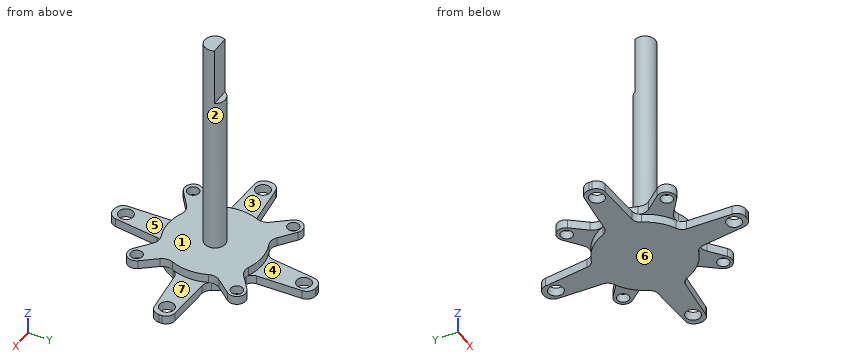
from build123d import *

# Parameters (mm, degrees)
SKETCH_2_R          = 3.5
EXTRUDE_1_DEPTH     = 75
SKETCH_3_R          = 2
EXTRUDE_2_DEPTH     = 3
FILLET_1_R          = 5
SKETCH_5_R          = 16
EXTRUDE_3_DEPTH     = 3
FILLET_2_R          = 4
SKETCH_6_R          = 2.5
EXTRUDE_4_DEPTH     = 3
FILLET_3_R          = 3
FILLET_4_R          = 3
CUT_EXTRUDE_1_DEPTH = 20


with BuildPart() as part:
    # 草图2 → 凸台-拉伸1 (new body)
    with BuildSketch(Plane.XY):
        Circle(SKETCH_2_R)
    extrude(amount=-EXTRUDE_1_DEPTH)

    # 草图3 → 凸台-拉伸2 (add)
    with BuildSketch(Plane(origin=(0, 0, -75), x_dir=(-1, 0, 0), z_dir=(0, 0, -1))):
        with BuildLine():
            Line((-19.333172355, 15.121758852), (-7.5, 0))
            Line((-7.5, 0), (-19.333172355, -15.121758852))
            ThreePointArc((-19.333172355, -15.121758852), (-19.091883092, -19.091883092), (-15.121758852, -19.333172355))
            Line((-15.121758852, -19.333172355), (0, -7.5))
            Line((0, -7.5), (15.407660085, -19.397223244))
            ThreePointArc((15.407660085, -19.397223244), (19.379165256, -19.127226562), (19.586420792, -15.151953404))
            Line((19.586420792, -15.151953404), (7.5, 0))
            Line((7.5, 0), (19.586420792, 15.151953404))
            ThreePointArc((19.586420792, 15.151953404), (19.379165256, 19.127226562), (15.407660085, 19.397223244))
            Line((15.407660085, 19.397223244), (0, 7.5))
            Line((0, 7.5), (-15.121758852, 19.333172355))
            ThreePointArc((-15.121758852, 19.333172355), (-19.091883092, 19.091883092), (-19.333172355, 15.121758852))
        make_face()
        with Locations((-16.970562748, 16.970562748)):
            Circle(SKETCH_3_R, mode=Mode.SUBTRACT)
        with Locations((16.970562748, 16.970562748)):
            Circle(SKETCH_3_R, mode=Mode.SUBTRACT)
        with Locations((16.970562748, -16.970562748)):
            Circle(SKETCH_3_R, mode=Mode.SUBTRACT)
        with Locations((-16.970562748, -16.970562748)):
            Circle(SKETCH_3_R, mode=Mode.SUBTRACT)
    extrude(amount=EXTRUDE_2_DEPTH)

    # 圆角1
    fillet_1_edges = [part.edges().sort_by_distance(p)[0] for p in [
        (7.5, 0, -76.5),
        (0, -7.5, -76.5),
        (-7.5, 0, -76.5),
        (0, 7.5, -76.5),
    ]]
    fillet(fillet_1_edges, radius=FILLET_1_R)

    # 草图5 → 凸台-拉伸3 (add)
    with BuildSketch(Plane.XY.offset(-75)):
        Circle(SKETCH_5_R)
    extrude(amount=-EXTRUDE_3_DEPTH)

    # 圆角2
    fillet_2_edges = [part.edges().sort_by_distance(p)[0] for p in [
        (8.070562783, -13.815426753, -76.5),
        (13.815426753, -8.070562783, -76.5),
        (-8.132091519, -13.779299239, -76.5),
        (-13.866910674, -7.981778521, -76.5),
        (-13.866910674, 7.981778521, -76.5),
        (-8.132091519, 13.779299239, -76.5),
        (8.070562783, 13.815426753, -76.5),
        (13.815426753, 8.070562783, -76.5),
    ]]
    fillet(fillet_2_edges, radius=FILLET_2_R)

    # 草图6 → 凸台-拉伸4 (add)
    with BuildSketch(Plane(origin=(0, 0, -78), x_dir=(-1, 0, 0), z_dir=(0, 0, -1))):
        with BuildLine():
            Line((-4.536268833, 32.087497482), (-5.241257707, 15.117182861))
            ThreePointArc((-5.241257707, 15.117182861), (-11.313708499, 11.313708499), (-15.117182861, 5.241257707))
            Line((-15.117182861, 5.241257707), (-32.087497482, 4.536268833))
            ThreePointArc((-32.087497482, 4.536268833), (-34.077297457, 3.667151814), (-34.959506593, 1.683121729))
            ThreePointArc((-34.959506593, 1.683121729), (-34.979209977, 1.206179654), (-34.992406887, 0.729013218))
            ThreePointArc((-34.992406887, 0.729013218), (-34.248960415, -1.311073956), (-32.323754723, -2.31519117))
            Line((-32.323754723, -2.31519117), (-15.442311817, -4.187482029))
            ThreePointArc((-15.442311817, -4.187482029), (-11.313708499, -11.313708499), (-4.187482029, -15.442311817))
            Line((-4.187482029, -15.442311817), (-2.31519117, -32.323754723))
            ThreePointArc((-2.31519117, -32.323754723), (-1.311073956, -34.248960415), (0.729013218, -34.992406887))
            ThreePointArc((0.729013218, -34.992406887), (1.206179654, -34.979209977), (1.683121729, -34.959506593))
            ThreePointArc((1.683121729, -34.959506593), (3.667151814, -34.077297457), (4.536268833, -32.087497482))
            Line((4.536268833, -32.087497482), (5.241257707, -15.117182861))
            ThreePointArc((5.241257707, -15.117182861), (11.313708499, -11.313708499), (15.117182861, -5.241257707))
            Line((15.117182861, -5.241257707), (32.087497482, -4.536268833))
            ThreePointArc((32.087497482, -4.536268833), (34.077297457, -3.667151814), (34.959506593, -1.683121729))
            ThreePointArc((34.959506593, -1.683121729), (34.979209977, -1.206179654), (34.992406887, -0.729013218))
            ThreePointArc((34.992406887, -0.729013218), (34.248960415, 1.311073956), (32.323754723, 2.31519117))
            Line((32.323754723, 2.31519117), (15.442311817, 4.187482029))
            ThreePointArc((15.442311817, 4.187482029), (11.313708499, 11.313708499), (4.187482029, 15.442311817))
            Line((4.187482029, 15.442311817), (2.31519117, 32.323754723))
            ThreePointArc((2.31519117, 32.323754723), (1.311073956, 34.248960415), (-0.729013218, 34.992406887))
            ThreePointArc((-0.729013218, 34.992406887), (-1.206179654, 34.979209977), (-1.683121729, 34.959506593))
            ThreePointArc((-1.683121729, 34.959506593), (-3.667151814, 34.077297457), (-4.536268833, 32.087497482))
        make_face()
        with Locations((-1.060660172, 30.759144982)):
            Circle(SKETCH_6_R, mode=Mode.SUBTRACT)
        with Locations(Location((30.759144982, -1.060660172, 0), (0, 0, 180))):
            Circle(SKETCH_6_R, mode=Mode.SUBTRACT)
        with Locations((1.060660172, -30.759144982)):
            Circle(SKETCH_6_R, mode=Mode.SUBTRACT)
        with Locations(Location((-30.759144982, 1.060660172, 0), (0, 0, 180))):
            Circle(SKETCH_6_R, mode=Mode.SUBTRACT)
    extrude(amount=EXTRUDE_4_DEPTH)

    # 圆角3
    # the kernel refuses this fillet: 3 mm, written as the material it adds along each edge
    with BuildSketch(Plane(origin=(5.241257707, 15.117182861, -78), x_dir=(0.9253660102129004, -0.379074856911743, 0), z_dir=(0, 0, -1))) as fillet_3_piece_1:
        with BuildLine():
            CenterArc((1.926011056, -2.995454288), FILLET_3_R, 93.154516435, 62.190253948)
            Line((-0.800492197, -1.743983149), (0, 0))
            ThreePointArc((0, 0), (0.880462197, -0.024243795), (1.760924394, 0))
        make_face()
    extrude(amount=3)

    # 圆角4
    # the kernel refuses this fillet: 3 mm, written as the material it adds along each edge
    with BuildSketch(Plane(origin=(15.117182861, 5.241257707, -78), x_dir=(-0.379074856911857, 0.9253660102128536, 0), z_dir=(0, 0, -1)), Plane(origin=(4.187482029, -15.442311817, -78), x_dir=(0.9492800359617337, 0.3144318898020519, 0), z_dir=(0, 0, -1)), Plane(origin=(-15.117182861, -5.241257707, -78), x_dir=(0.3790748569116308, -0.9253660102129463, 0), z_dir=(0, 0, -1)), Plane(origin=(-4.187482029, 15.442311817, -78), x_dir=(-0.9492800359616571, -0.3144318898022824, 0), z_dir=(0, 0, -1))) as fillet_4_piece_1:
        with BuildLine():
            CenterArc((1.926011056, 2.995454288), FILLET_4_R, 204.655229617, 62.190253948)
            Line((-0.800492197, 1.743983149), (0, 0))
            ThreePointArc((0, 0), (0.880462197, 0.024243795), (1.760924394, 0))
        make_face()
    extrude(amount=3)
    with BuildSketch(Plane(origin=(15.442311817, -4.187482029, -78), x_dir=(-0.314431889802168, -0.9492800359616952, 0), z_dir=(0, 0, -1))) as fillet_4_piece_2:
        with BuildLine():
            CenterArc((1.926011056, -2.995454288), FILLET_4_R, 93.154516435, 62.190253948)
            Line((-0.800492197, -1.743983149), (0, 0))
            ThreePointArc((0, 0), (0.880462197, -0.024243795), (1.760924394, 0))
        make_face()
    extrude(amount=3)
    with BuildSketch(Plane(origin=(-5.241257707, -15.117182861, -78), x_dir=(0.04150667502361383, -0.999138226637578, 0), z_dir=(0, 0, -1)), Plane(origin=(-15.442311817, 4.187482029, -78), x_dir=(-0.9939058470596024, -0.11023233273742473, 0), z_dir=(0, 0, -1))) as fillet_4_piece_3:
        with BuildLine():
            CenterArc((1.91892287, 3), FILLET_4_R, 207.809746052, 62.190253948)
            ThreePointArc((-0.734582019, 1.600388696), (-0.345257414, 0.810307818), (0, 0))
            Line((0, 0), (1.91892287, 0))
        make_face()
    extrude(amount=3)

    # 草图8 → 切除-拉伸1 (cut)
    with BuildSketch(Plane.XY):
        Polygon((-3.12402203, 1.578127484), (3.12402203, 1.578127484), (3.250549132, 4.217874186), (-3.12402203, 4.393016319), align=None)
    extrude(amount=-CUT_EXTRUDE_1_DEPTH, mode=Mode.SUBTRACT)


solid = part.part
Input: part model. Units: mm. Frame: model coordinates. Face numbers are marked on the shaded views. A direction names the side the tool comes from. Round coordinates to 2 decimals unless told otherwise and drop trailing zeros. Order: outer loops, then holes, each group sorted by start corner. A loop starts at its lowest first (then second) coordinate and runs counter-clockwise, first axis right, second up. Notation, with made-up numbers: (-17.5, 74.25) - (1.5, 74.25) arc R21 cw to (1.5, 82.25) - close; hole circle Ø4 at (39.25, 14). An arc over 180 degrees is marked (long way). Answer as a JSON object with one key per item and string values. Group by question number.
(1) Cut plane A-A (z = -72). Return loops of the section in (x, y), then the cut area to 3 significant figures.
(2) Material intervals for probe 1 along Z at (x, y) = (2.5, -21); probe 2 along Y at (x, z) = (0, -58.5); probe 3 along X at (y, z) = (2, -63), sorted ascending. Write a range as from..to.
(3) Pin query (flat end, axial travel): P1, Ø1.5, axis at x = 1.5, z = -23.5, coming from the +Y side; P2, Ø2, axis at x = -1, y = 2.5, coming from the +Z side; P3, Ø4, axis at x = 14, y = -11.5, coming from the -Z side; P4, Ø6, axis at y = 7.5, z = -16.5, coming from the -X side (3 decimals). Return the tip coordinate at first contact, or that it passes through.
(4) Draft query along Y for the marked faces 1, 2 and 3. Return one class per face: released by +Y, released by -Y, zero draft, split by the parting line, or undercut.
(5) Reachability of the marked faces 4, 5, 6 and 7 from +Z, -Z, +X, -X, +Y, -Y: full face, straight path, thin tool, end or side. Return the list, or none.
Here are the results:
{
 "1": {"outline": "circle Ø7 at (0, 0)", "area": "38.5 mm^2"},
 "2": {"probe 1": "z = -81..-78", "probe 2": "y = -3.5..3.5", "probe 3": "x = -2.87..2.87"},
 "3": {"P1": "stops at y = 3.42", "P2": "stops at z = 0", "P3": "stops at z = -78", "P4": "passes through"},
 "4": {"face 1": "zero draft", "face 2": "split by the parting line", "face 3": "undercut"},
 "5": {"face 4": "+Z, +Y", "face 5": "+Z, -Y", "face 6": "-Z, +X, -X, +Y, -Y", "face 7": "+Z, +X"}
}
